The model under review builds one solid part; all positions refer to its coordinate system, in mm. Face numbers are marked on the shaded views. A direction names the side the tool comes from. Coordinates: 2 decimals unless noted, no trailing zeros. Write each loop counter-clockwise with the first axis right and the second up, starting at its lowest first coordinate (ties: lowest second). Pieces come first, ordered by that corner, then holes. Notation, with made-up numbers: (68.25, -20.5) - (78.25, -20.5) arc R12 ccw to (78.25, -4.5) - close; hole circle Ø4 at (-26, 51). An arc over 180 degrees is marked (long way). Put each result on its own line as item: value. Start each with the question number.
Item 1: Mouldability with a two-part tool opening along Z and no side actions: class the marked faces 1, 2 and 3 as pulls with the +Z half, pulls with the -Z half, needs draft (parallel to the pull), parting line crosses it, or undercut.
Item 2: For pin 1 (4 mm diameter, centred on x = -52, z = 5, fed in from -Y); pin 2 (1.5 mm diameter, centred on x = -48, z = 1.5, fed in from -Y); pin 3 (3 mm diameter, centred on x = -48.5, y = -48.5, fed in from -Z); pin 4 (10 mm diameter, centred on x = -55, y = -27.5, fed in from +Z), all flat-tipped, find the tip position at first contact; note any pin that passes through.
Item 3: To check wall thickness, follow L1, parallel to Z at x = -49, y = -30.5; L2, parallel to Y at x = -45.75, z = 1; L3, parallel to Y at x = -47, z = 4.5. State the ranges of each line that lie inside material, in increasing order. Write a range as [from, to].
Item 4: Machinability: for the marked faces 4, 5 and 6, which of the approach directions +Z, -Z, +X, -X, +Y, -Y give a long, thin tool a straight path to every point of the face, cutting with its end or side? Answer none if there is none.
Item 5: Consider section B-B on x = -42. Give the boundary of the cut face in (y, z).
Item 6: Consider section C-C on y = -39. Give the boundary of the cut face in (x, z).
Item 7: Consider section D-D on x = -53.5. State how many separate pieces and enclosed holes the cut face has, then the cut area to 3 significant figures.
Item 8: Consider section A-A on z = 4. Give the boundary of the cut face in (x, y).
Solid Edge part; units mm, degrees
sketch "Sketch1" plane through (0, 0, 0) normal (0, 0, 1) x (1, 0, 0)
  circle A0 centre (-59.1628, -18.1899) radius 1
  line L0 (-40.0782, -20.6709) -> (-40.0782, -36.2909)
  arc A1 (-40.0782, -36.2909) -> (-41.0782, -37.2909) centre (-41.0782, -36.2909) cw
  line L1 (-41.0782, -37.2909) -> (-56.6982, -37.2909)
  line L2 (-60.5782, -33.4109) -> (-56.6982, -37.2909)
  line L3 (-60.5782, -33.4109) -> (-60.5782, -17.9909)
  arc A2 (-60.5782, -17.9909) -> (-59.3782, -16.7909) centre (-59.3782, -17.9909) cw
  line L4 (-59.3782, -16.7909) -> (-43.9582, -16.7909)
  line L5 (-43.9582, -16.7909) -> (-40.0782, -20.6709)
  circle A3 centre (-41.4332, -35.9309) radius 1
extrude "Protrusion1" add sketch "Sketch1" along normal blind 4.7
sketch "Sketch2" plane through (-50.3282, -27.0409, 4.7) normal (0, 0, 1) x (0, -1, 0)
  circle A0 centre (0, 0) radius 4.25
  arc A1 (-10.25, -3.9922) -> (-3.9922, -10.25) centre (0, 0) ccw
  line L0 (-3.9922, -10.25) -> (3.9922, -10.25)
  arc A2 (3.9922, -10.25) -> (10.25, -3.9922) centre (0, 0) ccw
  line L1 (10.25, 3.9922) -> (10.25, -3.9922)
  arc A3 (3.9922, 10.25) -> (10.25, 3.9922) centre (0, 0) cw
  line L2 (-3.9922, 10.25) -> (3.9922, 10.25)
  arc A4 (-3.9922, 10.25) -> (-10.25, 3.9922) centre (0, 0) ccw
  line L3 (-10.25, 3.9922) -> (-10.25, -3.9922)
extrude "ExtrudedProtrusion_2" add sketch "Sketch2" along normal blind 1.1
sketch "Sketch3" plane through (-50.3282, -27.0409, 5.8) normal (0, 0, 1) x (1, 0, 0)
  circle A0 centre (0, 0) radius 7
extrude "ExtrudedProtrusion_3" add sketch "Sketch3" along normal blind 1
sketch "Sketch4" plane through (-50.3282, -27.0409, 6.8) normal (0, 0, 1) x (1, 0, 0)
  circle A0 centre (0, 0) radius 2
extrude "ExtrudedProtrusion_4" add sketch "Sketch4" along normal blind 1.5
sketch "Sketch5" plane through (-50.3282, -27.0409, 8.3) normal (0, 0, 1) x (1, 0, 0)
  circle A0 centre (0, 0) radius 7
extrude "ExtrudedProtrusion_5" add sketch "Sketch5" along normal blind 2
sketch "Sketch6" plane through (-50.3282, 0, 0) normal (1, 0, 0) x (0, 1, 0)
  line L0 (-34.0409, 10.3) -> (-27.0409, 10.3)
  line L1 (-27.0409, 10.3) -> (-27.0409, 4.8545)
  arc A0 (-27.0409, 9.3) -> (-32.898, 10.0828) centre (-27.0409, 31.604) cw
  arc A1 (-32.898, 10.0828) -> (-34.0409, 9.1255) centre (-33.0685, 9.1255) ccw
  line L2 (-34.0409, 10.3) -> (-34.0409, 9.1255)
revolve "RevolvedCutout1" cut sketch "Sketch6" angle 360 about axis through (-50.3282, -27.0409, 10.3) along (0, 0, -1)
sketch "Sketch7" plane through (-48.8882, -37.2909, 2.9) normal (0, -1, 0) x (1, 0, 0)
  line L0 (-6.69, -0.7104) -> (-6.69, -2.7104)
  line L1 (-6.69, -2.7104) -> (3.81, -2.7104)
  line L2 (3.81, -2.7104) -> (3.81, -0.7104)
  line L3 (3.81, -0.7104) -> (-6.69, -0.7104)
extrude "ExtrudedProtrusion_6" add sketch "Sketch7" along normal blind 4
sketch "Sketch8" plane through (-50.3282, -39.2909, 0.1896) normal (0, 0, -1) x (0, -1, 0)
  line L0 (14, -1.25) -> (4.5, -1.25)
  line L1 (4.5, -1.25) -> (2, -5.25)
  line L2 (2, 5.25) -> (2, -5.25)
  line L3 (4.5, 1.25) -> (2, 5.25)
  line L4 (14, 1.25) -> (4.5, 1.25)
  line L5 (14, 0) -> (14, 1.25)
  line L6 (14, 0) -> (14, -1.25)
extrude "ExtrudedProtrusion_7" add sketch "Sketch8" against normal blind 0.1
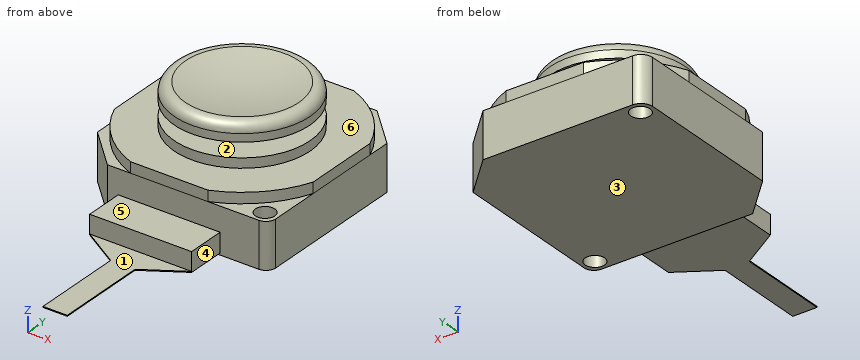
Report:
1. face 1: pulls with the +Z half
1. face 2: undercut
1. face 3: pulls with the -Z half
2. pin 1: y = -37.29
2. pin 2: y = -41.29
2. pin 3: z = 0.19
2. pin 4: z = 10.1
3. L1: [0, 4.7], [5.8, 6.8], [8.3, 9.61]
3. L2: [-41.29, -16.79]
3. L3: [-37.29, -16.79]
4. face 4: +Z, -Z, +X, -Y
4. face 5: +Z, +X, -X, -Y
4. face 6: +Z
5. outline: (-37.29, 0) - (-36.75, 0) - (-36.75, 4.7) - (-37.29, 4.7) - close; (-35.11, 0) - (-18.75, 0) - (-18.75, 4.7) - (-19.85, 4.7) - (-19.85, 5.8) - (-34.23, 5.8) - (-34.23, 4.7) - (-35.11, 4.7) - close
6. outline: (-55.58, 0.19) - (-45.08, 0.19) - (-45.08, 2.19) - (-55.58, 2.19) - close
7. separate pieces: 2
7. enclosed holes: 1
7. area: 151 mm²
8. outline: (-60.58, -33.41) - (-56.7, -37.29) - (-41.08, -37.29) arc R1 ccw to (-40.08, -36.29) - (-40.08, -20.67) - (-43.96, -16.79) - (-59.38, -16.79) arc R1.2 ccw to (-60.58, -17.99) - close; hole circle Ø2 at (-59.16, -18.19); hole circle Ø2 at (-41.43, -35.93)
